from build123d import *

# Parameters (mm, degrees)
F1_DEPTH = 25.4
F2_DEPTH = 6.35
F3_DEPTH = 25.4
F0_W     = 6.747447
F0_H     = 21.873236


with BuildPart() as f1:
    # F0 (on Front) → F1 (new body, symmetric)
    with BuildSketch(Plane.XZ):
        Polygon((36.823142, -9.641493), (36.823142, 9.641493), (25.886526, 9.641493), (-36.823142, 9.641493), (-36.823142, -9.641493), align=None)
    extrude(amount=F1_DEPTH, both=True)

    # F0 (on Front) → F2 (join, symmetric)
    with BuildSketch(Plane.XZ):
        with BuildLine():
            Line((-36.823142, 9.641493), (25.886526, 9.641493))
            Line((25.886526, 9.641493), (25.886526, 38.422067))
            ThreePointArc((25.886526, 38.422067), (30.875817, 50.467279), (42.921029, 55.456569))
            add(Edge.make_bspline(
                [(-36.823142, 9.641493), (-28.796567, 38.422067), (9.193794, 57.992861), (42.921029, 55.456569)],
                knots=[0, 0, 0, 0, 91.968223, 91.968223, 91.968223, 91.968223], degree=3))
        make_face()
    extrude(amount=F2_DEPTH, both=True)

    # F0 (on Front) → F3 (join, symmetric)
    with BuildSketch(Plane.XZ):
        with BuildLine():
            Line((25.886526, 9.641493), (36.823142, 9.641493))
            Line((36.823142, 9.641493), (36.823142, 38.422067))
            ThreePointArc((36.823142, 38.422067), (38.609172, 42.733923), (42.921029, 44.519953))
            Line((42.921029, 44.519953), (50.925627, 44.519953))
            Line((50.925627, 44.519953), (50.925627, 55.456569))
            Line((50.925627, 55.456569), (42.921029, 55.456569))
            ThreePointArc((42.921029, 55.456569), (30.875817, 50.467279), (25.886526, 38.422067))
            Line((25.886526, 38.422067), (25.886526, 9.641493))
        make_face()
    extrude(amount=F3_DEPTH, both=True)

    # F0 (on Front) → F4 (revolve)
    with BuildSketch(Plane.XZ):
        with Locations((72.303209, 50.509911)):
            Rectangle(F0_W, F0_H)
    revolve(axis=Axis((58.856271, 0, 50.509911), (0, 0, 1)))


solid = f1.part
Check sheet for the modelled part. Datum: model origin and axes. Units: mm. A direction names the side the tool comes from. Give positions to 0.01 mm unless a question says otherwise; leave off trailing zeros. Order: outer loops, then holes, each group sorted by start corner. A loop starts at its lowest first (then second) coordinate and runs counter-clockwise, first axis right, second up. Notation, with made-up numbers: (-40, 56.5) - (-6, 56.5) arc R16 cw to (-6, 68.5) - close; hole circle Ø3 at (-13.75, -26). An arc over 180 degrees is marked (long way). Answer as CSV lines item,"result".
1. Tool access check on faces 1 (the face through (50.926, -20, 50)), 2 (the face through (36.823, 0, 14)), 3 (the face through (25.887, 16, 24)), 4 (the face through (31.01, -16.01, 50.6)), 5 (the face through (50.926, 0, 50)). Record the directions out of +Z, -Z, +X, -X, +Y, -Y that give a thin tool (end or side, any length) a straight path to the whole face; none if there is none.
Result sheet:
face 1,"+Z, -Z, -Y"
face 2,"-Z, +X, +Y, -Y"
face 3,"+Z, -X, +Y"
face 4,"+Z, -X, -Y"
face 5,"+Z, -Z"
2. Scan lines: probe 1 along X at (y, z) = (-5, -5); probe 2 along Y at (x, z) = (-16.5, 27); probe 3 along Z at (x, y) = (-8.5, 15). Record each from-to range of solid material in increasing order. Write a range as from..to.
Result sheet:
probe 1,"-36.82..36.82"
probe 2,"-6.35..6.35"
probe 3,"-9.64..9.64"
3. Section check C-C (y = 11.5). Record the boundary of the cut face in (x, z).
Result sheet:
outline,"(-36.82, -9.64) - (36.82, -9.64) - (36.82, 38.42) arc R6.1 cw to (42.92, 44.52) - (46.58, 44.52) - (46.58, 39.57) - (71.13, 39.57) - (71.13, 61.45) - (46.58, 61.45) - (46.58, 55.46) - (42.92, 55.46) arc R17.03 ccw to (25.89, 38.42) - (25.89, 9.64) - (-36.82, 9.64) - close"
4. Section check A-A (y = 21.5). Record the boundary of the cut face in (x, z).
Result sheet:
outline,"(-36.82, -9.64) - (36.82, -9.64) - (36.82, 38.42) arc R6.1 cw to (42.92, 44.52) - (50.93, 44.52) - (50.93, 55.46) - (42.92, 55.46) arc R17.03 ccw to (25.89, 38.42) - (25.89, 9.64) - (-36.82, 9.64) - close"
5. Section check B-B (z = -1). Record the boundary of the cut face in (x, y), then the cut area to 3 significant figures.
Result sheet:
outline,"(-36.82, -25.4) - (36.82, -25.4) - (36.82, 25.4) - (-36.82, 25.4) - close"
area,"3,740 mm²"
6. Go/stop test with flat-tipped pins: P1, Ø10, axis at x = 64.5, y = -8, coming from the -Z side; P2, Ø8.5, axis at y = -2, z = 51.5, coming from the +X side; P3, Ø1, axis at y = 11.5, z = 23, coming from the -X side; P4, Ø3, axis at y = -19, z = 51, coming from the +X side. Record where each tip stops, or that it passes through.
Result sheet:
P1,"z = 39.57"
P2,"x = 75.68"
P3,"x = 25.89"
P4,"x = 50.93"
